Verification items for the finished model (mm, model axes). A direction names the side the tool comes from. Round coordinates to 2 decimals unless told otherwise and drop trailing zeros. Order: outer loops, then holes, each group sorted by start corner. A loop starts at its lowest first (then second) coordinate and runs counter-clockwise, first axis right, second up.
```python
from build123d import *

# Parameters (mm, degrees)
EXTRUDE_364_DEPTH   = 1.4
SKETCH_4_W          = 0.2
SKETCH_4_H          = 10.309401077
CHAMFER_2035_SIZE   = 0.32
FILLET_2080_R       = 0.1
SKETCH_7_R          = 1.592949274
CUT_EXTRUDE_1_DEPTH = 15


with BuildPart() as part:
    # 草图1 → Extrude 364 (new body)
    with BuildSketch(Plane(origin=(0, 0, 0), x_dir=(0, 0, -1), z_dir=(1, 0, 0))):
        Polygon((2, 1.154700538), (2, -1.154700538), (0, -2.309401077), (-2, -1.154700538), (-2, 1.154700538), (0, 2.309401077), align=None)
    extrude(amount=EXTRUDE_364_DEPTH)

    # 草图2 → 凸台-旋转1 (revolve)
    with BuildSketch(Plane.XY, mode=Mode.PRIVATE) as revolve_1_sk:
        Polygon((0, 0), (21.4, 0), (21.4, 0.6536), (21.4, 1), (7.791693541, 1), (0, 1), align=None)
    revolve(revolve_1_sk.sketch.rotate(Axis((0, 0, 0), (1, 0, 0)), 90), axis=Axis((0, 0, 0), (1, 0, 0)))

    # 草图3 → 切除-旋转1 (revolve, cut)
    with BuildSketch(Plane.XY):
        Polygon((0, 2), (3.065384141, 7.309401077), (3.065384141, 12.309401077), (-10, 12.309401077), (-10, 2), align=None)
    revolve(axis=Axis((0, 0, 0), (1, 0, 0)), mode=Mode.SUBTRACT)

    # 草图5 → 切除-旋转2 (revolve, cut)
    with BuildSketch(Plane.XY):
        Polygon((1.4, 2), (-1.665384141, 7.309401077), (-1.665384141, 12.309401077), (8.334615859, 12.309401077), (8.334615859, 2), align=None)
    revolve(axis=Axis((0, 0, 0), (1, 0, 0)), mode=Mode.SUBTRACT)

    # 草图4 → 切除-旋转3 (revolve, cut)
    with BuildSketch(Plane.XY, mode=Mode.PRIVATE) as cut_revolve_3_sk:
        with Locations((1.3, 7.154700539)):
            Rectangle(SKETCH_4_W, SKETCH_4_H)
    revolve(cut_revolve_3_sk.sketch.rotate(Axis((0, 0, 0), (1, 0, 0)), 270), axis=Axis((0, 0, 0), (1, 0, 0)), mode=Mode.SUBTRACT)

    # Chamfer 2035
    chamfer_2035_edges = [part.edges().sort_by_distance(p)[0] for p in [
        (21.4, 0, -1),
    ]]
    chamfer(chamfer_2035_edges, length=CHAMFER_2035_SIZE)

    # Fillet 2080
    fillet_2080_edges = [part.edges().sort_by_distance(p)[0] for p in [
        (1.4, 0, -1),
    ]]
    fillet(fillet_2080_edges, radius=FILLET_2080_R)

    # 草图7 → 切除-拉伸1 (cut)
    with BuildSketch(Plane(origin=(21.4, 0, 0), x_dir=(0, 0, -1), z_dir=(1, 0, 0))):
        Circle(SKETCH_7_R)
    extrude(amount=-CUT_EXTRUDE_1_DEPTH, mode=Mode.SUBTRACT)


solid = part.part
```
1) Go/stop test with flat-tipped pins: pin 1 Ø1 at (x, z) = (3, 1) entering from -Y; pin 2 Ø2 at (x, y) = (2.5, -1) entering from -Z; pin 3 Ø1.5 at (x, z) = (2, -0.5) entering from -Y. Record where each tip stops, or that it passes through.
2) Scan lines: probe 1 along X at (y, z) = (-0.65, -1.3); probe 2 along Y at (x, z) = (0.5, 0.8); probe 3 along Y at (x, z) = (1.75, -0.05). Record each from-to range of solid material in increasing order.
3) Tool access check on faces 1 (the flat face through (0.592, -1.724, -1.014)), 2 (the cylindrical face through (4, 1, 0)). Record the directions out of +Z, -Z, +X, -X, +Y, -Y that give a thin tool (end or side, any length) a straight path to the whole face; none if there is none.
4) Sectioned sample at A-A on x = 0.5. Record the cut outline in (y, z), then the cut area to 3 significant figures.
5) Sectioned sample at B-B on x = 3.25. Record the cut outline in (y, z).
Returned:
1. pin 1: stops at y = -0.87
1. pin 2: stops at z = -1
1. pin 3: stops at y = -2
2. probe 1: x = 0 to 1.4
2. probe 2: y = -1.85 to 1.85
2. probe 3: y = -1 to 1
3. face 1: -Z, +X, -X, -Y
3. face 2: +X
4. outline: (-2.31, 0) - (-1.15, -2) - (1.15, -2) - (2.31, 0) - (1.15, 2) - (-1.15, 2) - close
4. area: 13.9 mm2
5. outline: circle Ø2 at (0, 0)
